Autodesk Inventor part; units mm, degrees
ref_plane "Work Plane5" through (44.2715, 46.1721, 69.8769) normal (-1, 0, 0) x (0, 0, 1)
ref_plane "Work Plane7" through (57.0715, 40.1721, -25.6076) normal (-1, 0, 0) x (0, 0, 1)
ref_plane "YZ Plane" through (0, 0, 0) normal (1, 0, 0) x (0, 1, 0)
ref_plane "Work Plane1" through (49.1675, 65.1721, -19.9847) normal (0, 1, 0) x (-1, 0, 0)
sketch "Sketch1" plane through (49.1675, 65.1721, -19.9847) normal (0, 1, 0) x (-1, 0, 0)
  circle A0 centre (-2.8102, 4.1616) radius 0.75 construction
  circle A1 centre (-2.8102, 25.1616) radius 0.75 construction
  line L0 (11.6898, 12.5705) -> (11.6898, 16.7526) construction
  arc A2 (11.6898, 16.7526) -> (11.6898, 12.5705) centre (-2.8102, 14.6616) ccw construction
  arc A3 (6.4943, 19.8433) -> (3.1979, 23.455) centre (-2.8102, 14.6616) ccw construction
  arc A4 (3.1979, 5.8681) -> (6.3691, 9.2612) centre (-2.8102, 14.6616) ccw construction
  line L1 (6.4943, 19.8433) -> (10.0762, 19.8433) construction
  line L2 (10.0762, 19.8433) -> (10.0762, 9.2612) construction
  line L3 (10.0762, 9.2612) -> (6.3691, 9.2612) construction
  arc A5 (-8.8183, 23.455) -> (-8.8183, 5.8681) centre (-2.8102, 14.6616) ccw construction
  line L4 (15.1898, -17.3384) -> (-20.8102, -17.3384)
  line L5 (-20.8102, -17.3384) -> (-20.8102, 14.6616)
  line L6 (-20.8102, 14.6616) -> (15.1898, 14.6616)
  line L7 (15.1898, 14.6616) -> (15.1898, -17.3384)
  arc A6 (4.8861, 27.3616) -> (3.5031, 1.2204) centre (-2.8102, 14.6616) ccw construction
  line L8 (4.8861, 27.3616) -> (11.8898, 27.3616) construction
  line L9 (11.8898, 27.3616) -> (11.8898, 1.9616) construction
  line L10 (11.8898, 1.9616) -> (4.7096, 1.9616) construction
  line L11 (4.7096, 1.9616) -> (2.6908, 5.7766) construction
  arc A7 (2.6908, 5.7766) -> (6.254, 9.4612) centre (-2.8102, 14.6616) ccw construction
  line L12 (6.254, 9.4612) -> (9.8762, 9.4612) construction
  line L13 (9.8762, 9.4612) -> (9.8762, 19.6433) construction
  line L14 (9.8762, 19.6433) -> (6.376, 19.6433) construction
  arc A8 (6.376, 19.6433) -> (3.2687, 23.1616) centre (-2.8102, 14.6616) ccw construction
  line L15 (3.2687, 23.1616) -> (-8.889, 23.1616) construction
  arc A9 (-8.889, 23.1616) -> (-8.446, 5.8616) centre (-2.8102, 14.6616) ccw construction
  line L16 (-8.446, 5.8616) -> (1.0472, 5.8616) construction
  line L17 (1.0472, 5.8616) -> (3.5031, 1.2204) construction
  arc A10 (-17.6602, 14.6616) -> (4.7096, 1.9616) centre (-2.9041, 14.6019) ccw
  line L18 (4.7096, 1.9616) -> (11.8943, 1.9616)
  line L19 (11.8943, 1.9616) -> (11.8898, 14.6616)
  line L20 (11.8898, 14.6616) -> (15.1898, 14.6616)
  line L21 (3.1979, 5.8681) -> (-8.8183, 5.8681)
  line L22 (3.1979, 23.455) -> (-8.8183, 23.455)
  point P0 (49.1675, 19.9847)
  dimension "d0" = 32
  dimension "d2" = 18
  dimension "d3" = 18
  dimension "d4" = 0.2
extrude "Extrusion1" add sketch "Sketch1" against normal blind 15 contours L4 L5 L6 A10 L18 L19 L7
mirror "Mirror1" about plane through (37.2777, 65.1721, -5.3231) normal (0, 0, 1) of "Extrusion1"
sketch "Sketch4" plane through (33.9777, 50.1721, -37.3231) normal (-1, 0, 0) x (0, 0, 1)
  line L0 (0, 15) -> (64, 15)
  line L1 (0, 15) -> (0, 0)
  line L2 (0, 0) -> (64, 0)
  line L3 (64, 15) -> (64, 0)
  line L4 (0, 15) -> (64, 15)
  line L5 (64, 15) -> (88, 15)
  line L6 (88, 15) -> (88, 0)
  line L7 (88, 0) -> (64, 0)
  line L8 (64, 0) -> (64, 15)
  circle A0 centre (56, 7.5) radius 3
  circle A1 centre (56, 7.5) radius 5
  circle A2 centre (76, 7.5) radius 6
  point P0 (37.3231, -50.1721)
  dimension "d20" = 24
  dimension "d21" = 12
  dimension "d24" = 12
extrude "Extrusion4" add sketch "Sketch4" against normal up to surface (36 mm away) contours L5 L6 L7 L3
ref_plane "Work Plane4" through (33.9777, 57.6721, 36.6769) normal (1, 0, 0) x (0, 0, 1)
sketch "Sketch6" plane through (33.9777, 57.6721, 36.6769) normal (1, 0, 0) x (0, 0, 1)
  circle A0 centre (10, 0) radius 1.625 construction
  circle A1 centre (2, -8) radius 1.625
  circle A2 centre (-6, 0) radius 1.625 construction
  circle A3 centre (2, 8) radius 1.625
  circle A4 centre (2, 0) radius 4
  circle A5 centre (2, 0) radius 11 construction
  line L0 (14, 7.5) -> (-74, 7.5)
  arc A6 (10.0467, 7.5) -> (-6.0467, 7.5) centre (2, 0) ccw
  point P0 (-36.6769, 57.6721)
extrude "Extrusion6" add sketch "Sketch6" along normal blind 15 contours A3 L0 | A3 L0 A6 | L0 A3
sketch "Sketch5" plane through (33.9777, 50.1721, -37.3231) normal (-1, 0, 0) x (0, 0, 1)
  circle A0 centre (68, 7.5) radius 1.625
  circle A1 centre (84, 7.5) radius 1.625
  circle A2 centre (84, 7.5) radius 1.45
  circle A3 centre (68, 7.5) radius 1.45
  circle A4 centre (76, 15.5) radius 1.625
  circle A5 centre (76, -0.5) radius 1.625
  circle A6 centre (76, -0.5) radius 1.45
  circle A7 centre (76, 15.5) radius 1.45
  point P0 (37.3231, -50.1721)
  dimension "d25" = 2.9
  dimension "d26" = 2.9
  dimension "d31" = 2.9
  dimension "d32" = 2.9
extrude "Extrusion5" cut sketch "Sketch5" against normal blind 15 contours A2 | A3 | A6 | A7
sketch "Sketch7" plane through (33.9777, 50.1721, -37.3231) normal (-1, 0, 0) x (0, 0, 1)
  arc A0 (74.6389, 15) -> (77.3611, 15) centre (76, 15.5) ccw
  line L0 (0, 15) -> (74.6389, 15)
  line L1 (0, 15) -> (0, 0)
  line L2 (67.9533, 0) -> (0, 0)
  arc A1 (67.9533, 0) -> (84.0467, 0) centre (76, 7.5) ccw
  line L3 (88, 0) -> (84.0467, 0)
  line L4 (88, 15) -> (88, 0)
  line L5 (77.3611, 15) -> (88, 15)
  circle A2 centre (68, 7.5) radius 1.45
  circle A3 centre (84, 7.5) radius 1.45
  circle A4 centre (76, -0.5) radius 1.45
  circle A5 centre (76, 7.5) radius 6
  line L6 (0, 0) -> (88, 0)
  line L7 (88, 0) -> (106, 0)
  line L8 (106, 0) -> (106, 15)
  line L9 (106, 15) -> (88, 15)
  line L10 (88, 15) -> (88, 0)
  circle A6 centre (96, 7.5) radius 6.4305
  circle A7 centre (56, 7.5) radius 6.4532
  point P0 (37.3231, -50.1721)
  dimension "d34" = 20
  dimension "d35" = 10
  dimension "d40" = 20
extrude "Extrusion7" add sketch "Sketch7" against normal up to surface (36 mm away) contours L9 L8 L7 L4
sketch "Sketch9" plane through (33.9777, 50.1721, -37.3231) normal (-1, 0, 0) x (0, 0, 1)
  circle A0 centre (96, 7.5) radius 6.4305
  circle A1 centre (56, 7.5) radius 6.4506
  point P0 (37.3231, -50.1721)
  dimension "d41" = 40
extrude "Extrusion9" cut sketch "Sketch9" against normal through all contours A1
sketch "Sketch10" plane through (33.9777, 50.1721, 68.6769) normal (0, 0, 1) x (1, 0, 0)
  circle A0 centre (18.104, 4) radius 1.4
  circle A1 centre (18.104, 18) radius 1.4
  point P0 (-33.9777, -50.1721)
sketch "Sketch11" plane through (33.9777, 50.1721, -37.3231) normal (-1, 0, 0) x (0, 0, 1)
  circle A0 centre (114.9899, 4) radius 1.4
  circle A1 centre (114.9899, 18) radius 1.4
  line L0 (106, 15) -> (106, 0)
  line L1 (106, 0) -> (118, 0)
  line L2 (118, 0) -> (118, 22)
  line L3 (118, 22) -> (106, 22)
  line L4 (106, 22) -> (106, 0)
  circle A2 centre (114.9899, 4) radius 1.6
  circle A3 centre (114.9899, 18) radius 1.6
  point P0 (37.3231, -50.1721)
  dimension "d44" = 12
  dimension "d45" = 22
  dimension "d46" = 3.2
  dimension "d47" = 3.2
ref_plane "Work Plane5" through (44.2715, 46.1721, 69.8769) normal (-1, 0, 0) x (0, 0, 1)
extrude "Extrusion10" add sketch "Sketch11" against normal up to surface (10.2939 mm away) contours L4 L3 L2 L1 L0
sketch "Sketch12" plane through (49.1675, 50.1721, -19.9847) normal (0, -1, 0) x (1, 0, 0)
  circle A0 centre (-12.1429, -14.3384) radius 1.45
  circle A1 centre (-5.7536, -14.3384) radius 1.45
  circle A2 centre (-5.7536, -6.3384) radius 1.45
  circle A3 centre (11.5617, -14.3384) radius 1.45
  circle A4 centre (11.5617, -6.3384) radius 1.45
  circle A5 centre (17.951, -14.3384) radius 1.45
  circle A6 centre (10.8162, 47.0708) radius 1.45
  circle A7 centre (-5.0081, 47.0708) radius 1.45
  circle A8 centre (-10.0081, 47.0708) radius 1.45
  circle A9 centre (15.8162, 47.0708) radius 1.45
  circle A10 centre (2.9062, 47.0708) radius 1.45
  point P0 (-49.1675, 19.9847)
  dimension "d61" = 2.9
  dimension "d62" = 2.9
  dimension "d63" = 5
  dimension "d64" = 5
  dimension "d65" = 7.91
extrude "Extrusion11" cut sketch "Sketch12" against normal through all
sketch "Sketch13" plane through (49.1675, 50.1721, -19.9847) normal (0, -1, 0) x (1, 0, 0)
  arc A0 (-4.7096, 1.9616) -> (17.6602, 14.6616) centre (2.9041, 14.6019) ccw
  line L0 (-12.0959, -0.3981) -> (17.9041, -0.3981)
  line L1 (17.9041, -0.3981) -> (17.9041, 29.6019)
  line L2 (17.9041, 29.6019) -> (-12.0959, 29.6019)
  line L3 (-12.0959, 29.6019) -> (-12.0959, -0.3981)
  line L4 (-12.0959, -0.3981) -> (17.9041, 29.6019) construction
  line L5 (17.9041, -0.3981) -> (-12.0959, 29.6019) construction
  point P0 (-49.1675, 19.9847)
  dimension "d52" = 30
  dimension "d53" = 30
extrude "Extrusion12" cut sketch "Sketch13" against normal through all
chamfer "Chamfer1" distance 7 angle 45 2 edges at (52.0715, 50.1721, 9.6173) (52.0715, 50.1721, -20.3827)
ref_plane "Work Plane6" through (52.0715, 50.1721, -29.4723) normal (1, 0, 0) x (0, 1, 0)
sketch "Sketch14" plane through (52.0715, 50.1721, -29.4723) normal (1, 0, 0) x (0, 1, 0)
  line L0 (-2.0896, 10.3903) -> (12.6182, 10.3903)
  line L1 (12.6182, 10.3903) -> (12.6182, -2.343)
  line L2 (12.6182, -2.343) -> (-2.0896, -2.343)
  line L3 (-2.0896, -2.343) -> (-2.0896, 10.3903)
  point P0 (-50.1721, 29.4723)
ref_plane "Work Plane7" through (57.0715, 40.1721, -25.6076) normal (-1, 0, 0) x (0, 0, 1)
extrude "Extrusion14" cut sketch "Sketch14" along normal mid plane 30
properties part number "01_Slide_camera_x_v0"
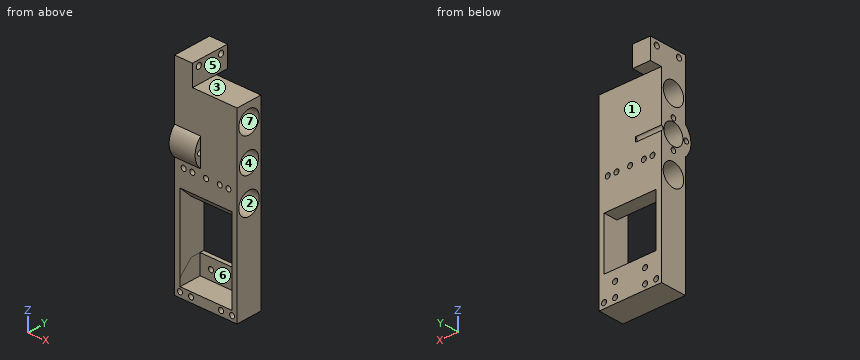
Work out the finished part from the listing and answer in its coordinate system (mm). Face numbers are marked on the shaded views. A direction names the side the tool comes from. Give positions to 0.01 mm unless a question says otherwise; leave off trailing zeros. Order: outer loops, then holes, each group sorted by start corner. A loop starts at its lowest first (then second) coordinate and runs counter-clockwise, first axis right, second up. Notation, with made-up numbers: (-7, 67) -> (40, 67) arc R26 ccw to (40, 90) -> close; hole circle Ø3 at (77.25, 23.5). An arc over 180 degrees is marked (long way). One line per item, written item: value.
Item 1: Find section C-C, the plane z = 23. Give the vertices of the cut face in (x, y).
Answer sheet:
outline: (33.98, 50.17) -> (69.98, 50.17) -> (69.98, 52.88) -> (33.98, 52.88) -> close; (33.98, 62.46) -> (69.98, 62.46) -> (69.98, 65.17) -> (33.98, 65.17) -> close
Item 2: Flat-ended cylindrical pins translate along their axes: P1, Ø4, axis at x = 52.5, y = 59, coming from the +Z side; P2, Ø12, axis at x = 50.5, y = 50, coming from the -Z side; P3, Ø1.7, axis at y = 57.67, z = 46.68, coming from the -X side; P4, Ø4.5, axis at x = 59.98, z = 27.09, coming from the +Y side. Find the tip coordinate at first contact, or state that the pin passes through.
Answer sheet:
P1: z = 68.68
P2: z = -37.32
P3: x = 48.98
P4: y = 65.17
Item 3: Straight lines are drawn through the part: probe 1 along Z at (x, y) = (47.5, 55); probe 2 along X at (y, z) = (62.75, -21); probe 3 along Z at (x, y) = (44, 65). For each, find the intervals that lie inside material, in ascending order.
Answer sheet:
probe 1: -37.32 to -31.82, 11.79 to 12.81, 24.55 to 33.3, 44.05 to 52.83, 64.53 to 68.68
probe 2: 33.98 to 37.07, 67.07 to 69.98
probe 3: -37.32 to -35.65, -33 to -27.65, -25 to -20.38, 9.62 to 25.64, 28.53 to 37.39, 39.96 to 80.68
Item 4: A tool of negligible diameter and unlimited length cuts with its end or side. For the marked faces 5, 6 and 7, from which of +Z, -Z, +X, -X, +Y, -Y can it reach the whole face along a straight path? Write none if from no direction.
Answer sheet:
face 5: +Z, +X, +Y, -Y
face 6: -Y
face 7: +X, -X
Item 5: Find section A-A, the plane z = -11. Give the vertices of the cut face in (x, y), plus the area to 3 significant figures.
Answer sheet:
outline: (33.98, 50.17) -> (37.07, 50.17) -> (37.07, 65.17) -> (33.98, 65.17) -> close; (67.07, 50.17) -> (69.98, 50.17) -> (69.98, 65.17) -> (67.07, 65.17) -> close
area: 90.0 mm²
Item 6: Determine the mould class of the marked faces 1, 2, 3 and 4 for opening direction Y: released by +Y, released by -Y, zero draft, split by the parting line, or undercut.
Answer sheet:
face 1: released by +Y
face 2: undercut
face 3: zero draft
face 4: undercut
Item 7: Find section B-B, the plane x = 57. Give the vertices of the cut face in (y, z).
Answer sheet:
outline: (50.17, -37.32) -> (65.17, -37.32) -> (65.17, -20.38) -> (62.79, -20.38) -> (62.79, -31.82) -> (50.17, -31.82) -> close; (50.17, 16.62) -> (57.17, 9.62) -> (65.17, 9.62) -> (65.17, 68.68) -> (50.17, 68.68) -> close; hole circle Ø12.9 at (57.67, 18.68); hole circle Ø12.86 at (57.67, 58.68); hole circle Ø12 at (57.67, 38.68)
